Design review of the part built by this model. Coordinates are the model's own, in mm. Face numbers are marked on the shaded views. A direction names the side the tool comes from. Coordinates: 2 decimals unless noted, no trailing zeros. Write each loop counter-clockwise with the first axis right and the second up, starting at its lowest first coordinate (ties: lowest second). Pieces come first, ordered by that corner, then holes. Notation, with made-up numbers: M -29.75,-5.5 L -1.75,-5.5 A13 cw -1.75,-1.5 Z; hole C -25,69.5 d8. An arc over 180 degrees is marked long. Return JSON: item names as keys, results as strings. Group by question number.
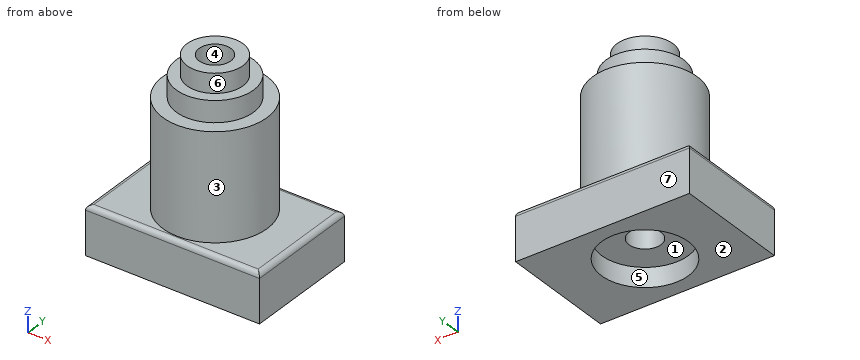
```python
from build123d import *

# Parameters (mm, degrees)
SKETCH_1_W          = 18
SKETCH_1_H          = 12
EXTRUDE_1_DEPTH     = 5
SKETCH_2_R          = 5.4
EXTRUDE_2_DEPTH     = 11
SKETCH_3_R          = 4
EXTRUDE_3_DEPTH     = 2.2
SKETCH_4_R          = 2.9
EXTRUDE_4_DEPTH     = 2
SKETCH_5_R          = 1.65
CUT_EXTRUDE_1_DEPTH = 25
SKETCH_6_R          = 4.5
CUT_EXTRUDE_2_DEPTH = 2
FILLET_1_R          = 0.5


with BuildPart() as part:
    # 草图1 → 凸台-拉伸1 (new body)
    with BuildSketch(Plane.XY):
        Rectangle(SKETCH_1_W, SKETCH_1_H)
    extrude(amount=EXTRUDE_1_DEPTH)

    # 草图2 → 凸台-拉伸2 (add)
    with BuildSketch(Plane.XY.offset(5)):
        Circle(SKETCH_2_R)
    extrude(amount=EXTRUDE_2_DEPTH)

    # 草图3 → 凸台-拉伸3 (add)
    with BuildSketch(Plane.XY.offset(16)):
        Circle(SKETCH_3_R)
    extrude(amount=EXTRUDE_3_DEPTH)

    # 草图4 → 凸台-拉伸4 (add)
    with BuildSketch(Plane.XY.offset(18.2)):
        Circle(SKETCH_4_R)
    extrude(amount=EXTRUDE_4_DEPTH)

    # 草图5 → 切除-拉伸1 (cut)
    with BuildSketch(Plane.XY.offset(20.2)):
        Circle(SKETCH_5_R)
    extrude(amount=-CUT_EXTRUDE_1_DEPTH, mode=Mode.SUBTRACT)

    # 草图6 → 切除-拉伸2 (cut)
    with BuildSketch(Plane(origin=(0, 0, 0), x_dir=(-1, 0, 0), z_dir=(0, 0, -1))):
        Circle(SKETCH_6_R)
    extrude(amount=-CUT_EXTRUDE_2_DEPTH, mode=Mode.SUBTRACT)

    # 圆角1
    fillet_1_edges = [part.edges().sort_by_distance(p)[0] for p in [
        (-9, 0, 5),
        (0, -6, 5),
        (9, 0, 5),
        (0, 6, 5),
    ]]
    fillet(fillet_1_edges, radius=FILLET_1_R)


solid = part.part
```
Item 1: For line 1 (Y direction, x = 0, z = 6.5); line 2 (Y direction, x = 0, z = 1); line 3 (Z direction, x = -6.25, y = 0.25), list the stretches that pass through material, from the lowest coordinate up.
Item 2: Machinability: for the marked faces 5, 6 and 7, which of the approach directions +Z, -Z, +X, -X, +Y, -Y give a long, thin tool a straight path to every point of the face, cutting with its end or side? Answer none if there is none.
Item 3: Add section D-D (x = -3.25). Write out the cut boundary in (y, z), plus the area to 3 significant figures.
Item 4: Add section A-A (x = 0). Write out the cut boundary in (y, z).
Item 5: Add section B-B (y = 0). Write out the cut boundary in (x, z).
Item 6: The part is to be moulded in two halves that separate along X. For the marked faces 1, 2, 3 and 4, say which applies: pulls with the +X half, pulls with the -X half, needs draft (parallel to the pull), parting line crosses it, or undercut.
Item 7: For pin 1 (1.5 mm diameter, centred on y = 3, z = 13, fed in from +X); pin 2 (1.5 mm diameter, centred on x = 2, y = -1, fed in from -Z), all flat-tipped, find the tip position at first contact; note any pin that passes through.
Item 8: Add section C-C (z = 2.25). Write out the cut boundary in (x, y).
Geometry check:
{
 "1": {"line 1": "-5.4 to -1.65, 1.65 to 5.4", "line 2": "-6 to -4.5, 4.5 to 6", "line 3": "0 to 5"},
 "2": {"face 5": "-Z", "face 6": "+Z", "face 7": "+Z, -Z, +X, -X, +Y"},
 "3": {"outline": "M -6,0 L -3.11,0 L -3.11,2 L 3.11,2 L 3.11,0 L 6,0 L 6,4.5 A0.5 ccw 5.5,5 L 4.31,5 L 4.31,16 L 2.33,16 L 2.33,18.2 L -2.33,18.2 L -2.33,16 L -4.31,16 L -4.31,5 L -5.5,5 A0.5 ccw -6,4.5 Z", "area": "153 mm^2"},
 "4": {"outline": "M -6,0 L -4.5,0 L -4.5,2 L -1.65,2 L -1.65,20.2 L -2.9,20.2 L -2.9,18.2 L -4,18.2 L -4,16 L -5.4,16 L -5.4,5 L -5.5,5 A0.5 ccw -6,4.5 Z; M 1.65,2 L 4.5,2 L 4.5,0 L 6,0 L 6,4.5 A0.5 ccw 5.5,5 L 5.4,5 L 5.4,16 L 4,16 L 4,18.2 L 2.9,18.2 L 2.9,20.2 L 1.65,20.2 Z"},
 "5": {"outline": "M -9,0 L -4.5,0 L -4.5,2 L -1.65,2 L -1.65,20.2 L -2.9,20.2 L -2.9,18.2 L -4,18.2 L -4,16 L -5.4,16 L -5.4,5 L -8.5,5 A0.5 ccw -9,4.5 Z; M 1.65,2 L 4.5,2 L 4.5,0 L 9,0 L 9,4.5 A0.5 ccw 8.5,5 L 5.4,5 L 5.4,16 L 4,16 L 4,18.2 L 2.9,18.2 L 2.9,20.2 L 1.65,20.2 Z"},
 "6": {"face 1": "undercut", "face 2": "needs draft", "face 3": "parting line crosses it", "face 4": "undercut"},
 "7": {"pin 1": "x = 4.91", "pin 2": "z = 2"},
 "8": {"outline": "M -9,-6 L 9,-6 L 9,6 L -9,6 Z; hole C 0,0 d3.3"}
}
